```python
from build123d import *

# Parameters (mm, degrees)
SKETCH1_W               = 55
SKETCH1_H               = 18
BOSS_EXTRUDE1_DEPTH     = 7.25
SHELL2_T                = 2
LENS_CUTOUT_REACH       = 38.517
POWER_BUTTON_HOLE_REACH = 38.517
SKETCH12_R              = 5
POWER_CORD_CUTOUT_REACH = 38.517
SKETCH13_W              = 8
SKETCH13_H              = 6
CUT_EXTRUDE4_DEPTH      = 37.517119273
FILLET4_R               = 2.5
BOSS_EXTRUDE3_DEPTH     = 2
M3_CLEARANCE_HOLE1_D    = 3.4
FILLET2_R               = 1
SKETCH18_W              = 2
SKETCH18_H              = 18.5
BOSS_EXTRUDE4_DEPTH     = 10
M3_CLEARANCE_HOLE2_D    = 3.4
FILLET3_R               = 2.5
FILLET5_R               = 4
FILLET6_R               = 1


with BuildPart() as part:
    # Sketch1 → Boss-Extrude1 (new, symmetric)
    with BuildSketch(Plane.XY):
        Rectangle(SKETCH1_W, SKETCH1_H)
    extrude(amount=BOSS_EXTRUDE1_DEPTH, both=True)

    # Shell2
    shell2_openings = [part.faces().sort_by_distance(p)[0] for p in [
        (0, 9, 0),
    ]]
    offset(amount=SHELL2_T, openings=shell2_openings, kind=Kind.INTERSECTION)

    # Sketch11 → lens cutout (cut, up to next)
    with BuildSketch(Plane.XY.offset(9.25), mode=Mode.PRIVATE) as lens_cutout_sk1:
        with BuildLine():
            Line((-27.5, 9), (-27.5, 1))
            ThreePointArc((-27.5, 1), (-17.5, -9), (-7.5, 1))
            Line((-7.5, 1), (-7.5, 9))
            Line((-7.5, 9), (-27.5, 9))
        make_face()
    lens_cutout_tool1 = extrude(lens_cutout_sk1.sketch, amount=-LENS_CUTOUT_REACH, mode=Mode.PRIVATE) & part.part
    add(lens_cutout_tool1.solids().sort_by_distance((-17.5, 0.915899, 9.25))[0], mode=Mode.SUBTRACT)

    # Sketch12 → power button hole (cut, up to next)
    with BuildSketch(Plane.XY.offset(9.25), mode=Mode.PRIVATE) as power_button_hole_sk1:
        with Locations((13.5, 1)):
            Circle(SKETCH12_R)
    power_button_hole_tool1 = extrude(power_button_hole_sk1.sketch, amount=-POWER_BUTTON_HOLE_REACH, mode=Mode.PRIVATE) & part.part
    add(power_button_hole_tool1.solids().sort_by_distance((13.5, 1, 9.25))[0], mode=Mode.SUBTRACT)

    # Sketch13 → power cord cutout (cut, up to next)
    with BuildSketch(Plane(origin=(0, 0, -9.25), x_dir=(-1, 0, 0), z_dir=(0, 0, -1)), mode=Mode.PRIVATE) as power_cord_cutout_sk1:
        with Locations((-15.5, 6)):
            Rectangle(SKETCH13_W, SKETCH13_H)
    power_cord_cutout_tool1 = extrude(power_cord_cutout_sk1.sketch, amount=-POWER_CORD_CUTOUT_REACH, mode=Mode.PRIVATE) & part.part
    add(power_cord_cutout_tool1.solids().sort_by_distance((15.5, 6, -9.25))[0], mode=Mode.SUBTRACT)

    # Sketch21 → Cut-Extrude4 (cut, through all)
    with BuildSketch(Plane.XY.offset(9.25)):
        with BuildLine():
            Line((-3.5, 7), (3.5, 7))
            ThreePointArc((3.5, 7), (5, 5.5), (3.5, 4))
            Line((3.5, 4), (-3.5, 4))
            ThreePointArc((-3.5, 4), (-5, 5.5), (-3.5, 7))
        make_face()
    extrude(amount=-CUT_EXTRUDE4_DEPTH, mode=Mode.SUBTRACT)

    # Fillet4
    fillet4_edges = [part.edges().sort_by_distance(p)[0] for p in [
        (-7.5, 9, 8.25),
    ]]
    fillet(fillet4_edges, radius=FILLET4_R)

    # Sketch15 → Boss-Extrude3 (add)
    with BuildSketch(Plane.XZ.offset(11)):
        Polygon((-29.5, 9.25), (-29.5, -9.25), (-36, -11.96461114), (-36, 6.53538886), align=None)
    extrude(amount=-BOSS_EXTRUDE3_DEPTH)

    # M3 Clearance Hole1 (through all)
    with Locations(Plane(origin=(0, -9, 0), x_dir=(1, 0, 0), z_dir=(0, 1, 0))):
        with Locations((-32.75, 1.35730557)):
            Hole(M3_CLEARANCE_HOLE1_D / 2)

    # Fillet2
    fillet2_edges = [part.edges().sort_by_distance(p)[0] for p in [
        (-29.5, -9, 0),
    ]]
    fillet(fillet2_edges, radius=FILLET2_R)

    # Sketch18 → Boss-Extrude4 (add)
    with BuildSketch(Plane.XZ.offset(11)):
        with Locations((28.5, 0)):
            Rectangle(SKETCH18_W, SKETCH18_H)
    extrude(amount=BOSS_EXTRUDE4_DEPTH)

    # M3 Clearance Hole2 (through all)
    with Locations(Plane.ZY.offset(-27.5)):
        with Locations((-4.5, -17), (4.5, -17)):
            Hole(M3_CLEARANCE_HOLE2_D / 2)

    # Fillet3
    fillet3_edges = [part.edges().sort_by_distance(p)[0] for p in [
        (27.5, -11, 0),
    ]]
    fillet(fillet3_edges, radius=FILLET3_R)

    # Fillet5
    fillet5_edges = [part.edges().sort_by_distance(p)[0] for p in [
        (-28.5, 9, 9.25),
    ]]
    fillet(fillet5_edges, radius=FILLET5_R)

    # Fillet6
    fillet6_edges = [part.edges().sort_by_distance(p)[0] for p in [
        (-36, -10, 6.53538886),
        (-36, -10, -11.96461114),
        (28.5, -21, 9.25),
        (28.5, -21, -9.25),
    ]]
    fillet(fillet6_edges, radius=FILLET6_R)


solid = part.part
```
Can you work these out from the model? Positions are in its coordinate system, mm. A direction names the side the tool comes from. Give positions to 0.01 mm unless a question says otherwise; leave off trailing zeros. Write each loop counter-clockwise with the first axis right and the second up, starting at its lowest first coordinate (ties: lowest second). Pieces come first, ordered by that corner, then holes. Notation, with made-up numbers: (84.5, 37) -> (139.5, 37) arc R31 ccw to (139.5, 66) -> close; hole circle Ø3 at (-14.75, -35.75). An arc over 180 degrees is marked (long way). Write item = value, one per line.
(1) Thinking about a two-plate mould opening in Z: for faces 6 (the face through (28, -21, 0)), 7 (the face through (28.51, -16.49, -6.12)), 8 (the face through (6, -2, 9.25)), which applies, released by +Z, released by -Z, zero draft, split by the parting line, or undercut?
Worked out:
face_6 = zero draft
face_7 = undercut
face_8 = released by +Z
(2) Suppose I cut it at C-C on y = -1.75. Write out the boundary of the cut face in (x, z).
Worked out:
outline = (-29.5, -9.25) -> (29.5, -9.25) -> (29.5, 9.25) -> (17.68, 9.25) -> (17.68, 7.25) -> (27.5, 7.25) -> (27.5, -7.25) -> (-27.5, -7.25) -> (-27.5, 7.25) -> (-27.11, 7.25) -> (-27.11, 9.25) -> (-29.5, 9.25) -> close; (-7.89, 7.25) -> (9.32, 7.25) -> (9.32, 9.25) -> (-7.89, 9.25) -> close
(3) Suppose I cut it at D-D on x = -8.5. Write out the boundary of the cut face in (y, z).
Worked out:
outline = (-11, -9.25) -> (9, -9.25) -> (9, -7.25) -> (-9, -7.25) -> (-9, 7.25) -> (-3.36, 7.25) -> (-3.36, 9.25) -> (-11, 9.25) -> close
(4) Suppose I cut it at A-A on y = -17. Write out the boundary of the cut face in (x, z).
Worked out:
outline = (27.5, -9.25) -> (29.5, -9.25) -> (29.5, -6.2) -> (27.5, -6.2) -> close; (27.5, -2.8) -> (29.5, -2.8) -> (29.5, 2.8) -> (27.5, 2.8) -> close; (27.5, 6.2) -> (29.5, 6.2) -> (29.5, 9.25) -> (27.5, 9.25) -> close
(5) For faces 1 (the face through (0, 4, -8)), 2 (the face through (-5, -11, -1)), 3 (the face through (-29.5, 0, 0)), 4 (the face through (16, 3, -8)), 5 (the face through (27.5, 0, 0)), which set-ups out of +Z, -Z, +X, -X, +Y, -Y let a thin tool reach every point of the face, with its end or its side?
Worked out:
face_1 = +Z, -Z
face_2 = +Z, -Z, -X, -Y
face_3 = +Z, -Z, -X, +Y
face_4 = -Z, +Y
face_5 = +Y
(6) I'm going to push flat-ended pins straight in: P1, Ø2, axis at y = -15.5, z = 3.5, coming from the -X side; P2, Ø3, axis at x = -25, y = -3.5, coming from the -Z side; P3, Ø1, axis at y = 4.5, z = -8.5, coming from the -X side. Where does each tip first touch, or does it pass through?
Worked out:
P1 = 27.5
P2 = -9.25
P3 = -29.5
(7) Suppose I cut it at B-B on z = 4.5. Write out the boundary of the cut face in (x, y).
Worked out:
outline = (-36, -11) -> (25, -11) arc R2.5 cw to (27.5, -13.5) -> (27.5, -15.3) -> (29.5, -15.3) -> (29.5, 9) -> (27.5, 9) -> (27.5, -9) -> (-27.5, -9) -> (-27.5, 9) -> (-29.5, 9) -> (-29.5, -8) arc R1 cw to (-30.5, -9) -> (-36, -9) -> close; (27.5, -21) -> (29.5, -21) -> (29.5, -18.7) -> (27.5, -18.7) -> close
(8) I need wall thicknesses on probe 1 along Y at (x, z) = (28.1, 4.5); probe 2 along Z at (x, y) = (-9, -8); probe 3 along X at (y, z) = (-7.5, -6.75). Which ranges of each line are inside material? Lowest first, please. Write a range as from..to.
Worked out:
probe_1 = -21..-18.7, -15.3..9
probe_2 = -9.25..-7.25, 7.25..9.25
probe_3 = -29.5..-27.5, 27.5..29.5
